Read the model definition and answer for the solid it produces. Units are mm, in the model's axes. A direction names the side the tool comes from. Coordinates: 2 decimals unless noted, no trailing zeros. Loops run counter-clockwise (first coordinate to the right, second up) from the corner with the lowest first, then second, coordinate; pieces in that order, holes last. Notation, with made-up numbers: M -32,39 L 13,39 A15 cw 13,52 Z; hole C -9.75,86.25 d2. An arc over 180 degrees is marked long. Use one line per item in the form item = value. Start each with the question number.
1. The part is cut by section C-C (x = 98.5). Give the vertices of the cut face in (y, z), plus the area to 3 significant figures.
2. Flat-ended cylindrical pins translate along their axes: pin 1 (1.5 mm diameter, centred on x = 90, y = 4.5, fed in from +Z); pin 2 (1.3 mm diameter, centred on x = 150, z = 8, fed in from -Y); pin 3 (10 mm diameter, centred on x = 147.5, z = -1, fed in from -Y). Find the tip coordinate at first contact, or state that the pin passes through.
3. Find the intervals of material crossed by probe 1 along Z at (x, y) = (150, 3.8); probe 2 along X at (y, z) = (3.5, -12); probe 3 along Z at (x, y) = (116, 1.25), in increasing order. Write a range as [from, to].
4. A tool of negligible diameter and unlimited length cuts with its end or side. For faces 4 (the flat face through (70.6, 5.22, -1.94)), 5 (the flat face through (152.5, 3, -2)), from which of +Z, -Z, +X, -X, +Y, -Y can it reach the whole face along a straight path? Write none if from no direction.
5. For a pull along X with two mould halves and no side action, classify faces 1 (the flat face through (146, 1.46, -2)), 2 (the flat face through (96.99, 5.22, -1.94)), 3 (the cylindrical face through (148.95, 2.98, 7.95)) as released by +X, released by -X, zero draft, split by the parting line, or undercut.
6. The part is cut by section A-A (x = 150). Give the vertices of the cut face in (y, z).
7. The part is cut by section B-B (z = 8). Give the vertices of the cut face in (x, y).
from build123d import *

# Parameters (mm, degrees)
BOSS_EXTRU_1_DEPTH      = 8
ESQUISSE3_W             = 25
ESQUISSE3_H             = 3
BOSS_EXTRU_3_DEPTH      = 12.5
ESQUISSE4_R             = 1.05
ENL_V_MAT_EXTRU_1_DEPTH = 10
ESQUISSE7_W             = 13.702754964
ESQUISSE7_H             = 7.283651796
ENL_V_MAT_EXTRU_2_DEPTH = 55


with BuildPart() as part:
    # Esquisse1 → Boss.-Extru.1 (new body)
    with BuildSketch(Plane.XY.offset(2)):
        Polygon((55.971983753, 0), (140, 0), (140, 4.46), (139.050191247, 4.46), (138.489677086, 6), (137.899678914, 6), (137.339164753, 4.46), (136.851078247, 4.46), (136.290564086, 6), (135.700565914, 6), (135.140051753, 4.46), (134.651965247, 4.46), (134.091451086, 6), (133.501452914, 6), (132.940938753, 4.46), (132.452852247, 4.46), (131.892338086, 6), (131.302339914, 6), (130.741825753, 4.46), (130.253739247, 4.46), (129.693225086, 6), (129.103226914, 6), (128.542712753, 4.46), (128.054626247, 4.46), (127.494112086, 6), (126.904113914, 6), (126.343599753, 4.46), (125.855513247, 4.46), (125.294999086, 6), (124.705000914, 6), (124.144486753, 4.46), (123.656400247, 4.46), (123.095886086, 6), (122.505887914, 6), (121.945373753, 4.46), (121.457287247, 4.46), (120.896773086, 6), (120.306774914, 6), (119.746260753, 4.46), (119.258174247, 4.46), (118.697660086, 6), (118.107661914, 6), (117.547147753, 4.46), (117.059061247, 4.46), (116.498547086, 6), (115.908548914, 6), (115.348034753, 4.46), (114.859948247, 4.46), (114.299434086, 6), (113.709435914, 6), (113.148921753, 4.46), (112.660835247, 4.46), (112.100321086, 6), (111.510322914, 6), (110.949808753, 4.46), (110.461722247, 4.46), (109.901208086, 6), (109.311209914, 6), (108.750695753, 4.46), (108.262609247, 4.46), (107.702095086, 6), (107.112096914, 6), (106.551582753, 4.46), (106.063496247, 4.46), (105.502982086, 6), (104.912983914, 6), (104.352469753, 4.46), (103.864383247, 4.46), (103.303869086, 6), (102.713870914, 6), (102.153356753, 4.46), (101.665270247, 4.46), (101.104756086, 6), (100.514757914, 6), (99.954243753, 4.46), (99.466157247, 4.46), (98.905643086, 6), (98.315644914, 6), (97.755130753, 4.46), (97.267044247, 4.46), (96.706530086, 6), (96.116531914, 6), (95.556017753, 4.46), (95.067931247, 4.46), (94.507417086, 6), (93.917418914, 6), (93.356904753, 4.46), (92.868818247, 4.46), (92.308304086, 6), (91.718305914, 6), (91.157791753, 4.46), (90.669705247, 4.46), (90.109191086, 6), (89.519192914, 6), (88.958678753, 4.46), (88.470592247, 4.46), (87.910078086, 6), (87.320079914, 6), (86.759565753, 4.46), (86.271479247, 4.46), (85.710965086, 6), (85.120966914, 6), (84.560452753, 4.46), (84.072366247, 4.46), (83.511852086, 6), (82.921853914, 6), (82.361339753, 4.46), (81.873253247, 4.46), (81.312739086, 6), (80.722740914, 6), (80.162226753, 4.46), (79.674140247, 4.46), (79.113626086, 6), (78.523627914, 6), (77.963113753, 4.46), (77.475027247, 4.46), (76.914513086, 6), (76.324514914, 6), (75.764000753, 4.46), (75.275914247, 4.46), (74.715400086, 6), (74.125401914, 6), (73.564887753, 4.46), (73.076801247, 4.46), (72.516287086, 6), (71.926288914, 6), (71.365774753, 4.46), (70.877688247, 4.46), (70.317174086, 6), (69.727175914, 6), (69.166661753, 4.46), (68.678575247, 4.46), (68.118061086, 6), (67.528062914, 6), (66.967548753, 4.46), (66.479462247, 4.46), (65.918948086, 6), (65.328949914, 6), (64.768435753, 4.46), (64.280349247, 4.46), (63.719835086, 6), (63.129836914, 6), (62.569322753, 4.46), (62.081236247, 4.46), (61.520722086, 6), (60.930723914, 6), (60.370209753, 4.46), (59.882123247, 4.46), (59.321609086, 6), (58.731610914, 6), (58.171096753, 4.46), (57.683010247, 4.46), (57.122496086, 6), (56.532497914, 6), (55.971983753, 4.46), align=None)
    extrude(amount=-BOSS_EXTRU_1_DEPTH)

    # Esquisse3 → Boss.-Extru.3 (add)
    with BuildSketch(Plane(origin=(140, 0, 0), x_dir=(0, 0, -1), z_dir=(1, 0, 0))):
        with Locations((2, 2.96)):
            Rectangle(ESQUISSE3_W, ESQUISSE3_H)
    extrude(amount=BOSS_EXTRU_3_DEPTH)

    # Esquisse4 → Enlèv. mat.-Extru.1 (cut)
    with BuildSketch(Plane(origin=(0, 4.46, 0), x_dir=(1, 0, 0), z_dir=(0, 1, 0))):
        with Locations((150, -8)):
            Circle(ESQUISSE4_R)
        with Locations((150, 12)):
            Circle(ESQUISSE4_R)
    extrude(amount=-ENL_V_MAT_EXTRU_1_DEPTH, mode=Mode.SUBTRACT)

    # Esquisse7 → Enlèv. mat.-Extru.2 (cut)
    with BuildSketch(Plane(origin=(152.5, 0, 0), x_dir=(0, 0, -1), z_dir=(1, 0, 0))):
        with Locations((2.202713729, 8.101825898)):
            Rectangle(ESQUISSE7_W, ESQUISSE7_H)
    extrude(amount=-ENL_V_MAT_EXTRU_2_DEPTH, mode=Mode.SUBTRACT)


solid = part.part
Computed values:
q1.outline = M 0,-6 L 4.46,-6 L 4.46,2 L 0,2 Z
q1.area = 35.7 mm²
q2.pin_1 = 2
q2.pin_2 = through
q2.pin_3 = 1.46
q3.probe_1 = [-14.5, -13.05], [-10.95, 6.95], [9.05, 10.5]
q3.probe_2 = [140, 148.95], [151.05, 152.5]
q3.probe_3 = [-6, 2]
q4.face_4 = +Z, -Z, +Y
q4.face_5 = +Z, -Z, +X, +Y, -Y
q5.face_1 = zero draft
q5.face_2 = released by +X
q5.face_3 = undercut
q6.outline = M 1.46,-14.5 L 4.46,-14.5 L 4.46,-13.05 L 1.46,-13.05 Z; M 1.46,-10.95 L 4.46,-10.95 L 4.46,6.95 L 1.46,6.95 Z; M 1.46,9.05 L 4.46,9.05 L 4.46,10.5 L 1.46,10.5 Z
q7.outline = M 140,1.46 L 148.95,1.46 L 148.95,4.46 L 140,4.46 Z; M 151.05,1.46 L 152.5,1.46 L 152.5,4.46 L 151.05,4.46 Z
